Design review of the part built by this model. Coordinates are the model's own, in mm. Coordinates: 2 decimals unless noted, no trailing zeros. Loops run counter-clockwise (first coordinate to the right, second up) from the corner with the lowest first, then second, coordinate; pieces in that order, holes last. Notation, with made-up numbers: (74, -6.75) -> (133, -6.75) arc R23 ccw to (133, 31.25) -> close; hole circle Ø6 at (19, 37.5). An arc over 180 degrees is marked (long way). Answer as a JSON object with one key per item and string values.
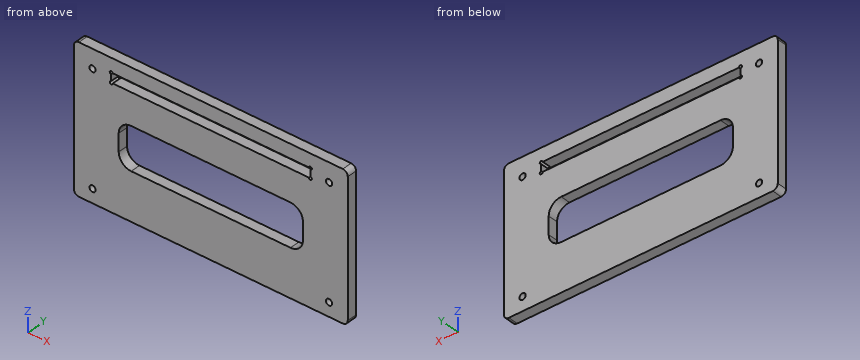
Autodesk Inventor part; units mm, degrees
ref_plane "YZ Plane" through (0, 0, 0) normal (1, 0, 0) x (0, 1, 0)
ref_plane "XZ Plane" through (0, 0, 0) normal (0, 1, 0) x (-1, 0, 0)
ref_plane "XY Plane" through (0, 0, 0) normal (0, 0, 1) x (1, 0, 0)
sketch "Sketch1" plane through (0, 0, 0) normal (0, 1, 0) x (-1, 0, 0)
  line L0 (55, -28) -> (-55, -28)
  line L1 (-55, -28) -> (-55, 28)
  line L2 (-55, 28) -> (55, 28) construction
  line L3 (55, 28) -> (55, -28)
  circle A0 centre (47.5, -22.5) radius 1.25
  circle A1 centre (-47.5, -22.5) radius 1.25
  circle A2 centre (-47.5, 22.5) radius 1.25
  circle A3 centre (47.5, 22.5) radius 1.25
  line L4 (47.5, -22.5) -> (-47.5, -22.5) construction
  line L5 (-47.5, -22.5) -> (-47.5, 22.5) construction
  line L6 (-32, -9) -> (32, -9)
  line L7 (32, 8) -> (-32, 8)
  line L8 (-55, 28) -> (-55, 30)
  line L9 (-55, 30) -> (55, 30)
  line L10 (55, 30) -> (55, 28)
  line L11 (37, 3) -> (37, -4)
  line L12 (-37, 3) -> (-37, -4)
  arc A4 (37, 3) -> (32, 8) centre (32, 3) ccw
  arc A5 (32, -9) -> (37, -4) centre (32, -4) ccw
  arc A6 (-32, 8) -> (-37, 3) centre (-32, 3) ccw
  arc A7 (-37, -4) -> (-32, -9) centre (-32, -4) ccw
  point P0 (0, 0)
  point P1 (-55, 0)
  point P2 (0, 28)
  point P3 (-47.5, 0)
  point P4 (0, -22.5)
  point P5 (-37, -9)
  point P6 (37, -9)
  point P7 (37, 8)
  point P8 (-37, 8)
  point P9 (0, 8)
  dimension "d0" = 110
  dimension "d1" = 56
  dimension "d2" = 2.5
  dimension "d3" = 95
  dimension "d4" = 45
  dimension "d18" = 2
  dimension "d20" = 74
  dimension "d21" = 19
  dimension "d22" = 17
  dimension "d23" = 5
extrude "Extrusion1" add sketch "Sketch1" along normal mid plane 4
fillet "Fillet1" radius 2 4 edges at (55, 0, -28) (-55, 0, -28) (-55, 0, 30) (55, 0, 30)
sketch "Sketch2" plane through (0, 2, 0) normal (0, 1, 0) x (1, 0, 0)
  line L0 (-40, -20.65) -> (-39.4, -20.65) construction
  line L1 (40, -20.65) -> (40, -21.25) construction
  line L2 (40, -24.45) -> (39.4, -24.45) construction
  line L3 (-40, -24.45) -> (-40, -23.85) construction
  arc A0 (-40, -23.85) -> (-39.4, -24.45) centre (-40, -24.45) ccw
  arc A1 (-39.4, -20.65) -> (-40, -21.25) centre (-40, -20.65) ccw
  arc A2 (40, -21.25) -> (39.4, -20.65) centre (40, -20.65) ccw
  arc A3 (39.4, -24.45) -> (40, -23.85) centre (40, -24.45) ccw
  line L4 (-40, -23.85) -> (-40, -21.25)
  line L5 (-39.4, -24.45) -> (-40, -24.45) construction
  arc A4 (-40, -21.25) -> (-39.4, -20.65) centre (-40, -20.65) ccw construction
  line L6 (-40, -21.25) -> (-40, -20.65) construction
  line L7 (-39.4, -20.65) -> (39.4, -20.65)
  line L8 (39.4, -24.45) -> (-39.4, -24.45)
  line L9 (40, -23.85) -> (40, -24.45) construction
  arc A5 (40, -23.85) -> (39.4, -24.45) centre (40, -24.45) ccw construction
  arc A6 (39.4, -20.65) -> (40, -21.25) centre (40, -20.65) ccw construction
  line L10 (40, -21.25) -> (40, -23.85)
  line L11 (39.4, -20.65) -> (40, -20.65) construction
  line L12 (-53, -30) -> (53, -30)
  point P0 (0, 0)
  point P1 (0, -24.45)
  dimension "d9" = 3.8
  dimension "d11" = 80
  dimension "d14" = 1.2
  dimension "d19" = 5.55
extrude "Extrusion2" cut sketch "Sketch2" against normal through all
properties part number "Marco conectores IC DC" material "Polycarbonate, Smoke"
1) Add section C-C, the plane z = 22.5. Give the boundary of the cut face in (x, y), and give its area (3 significant figures).
Completed:
{"outline": "(-55, -2) -> (-48.75, -2) -> (-48.75, 2) -> (-55, 2) -> close; (-46.25, -2) -> (-40, -2) -> (-40, 2) -> (-46.25, 2) -> close; (40, -2) -> (46.25, -2) -> (46.25, 2) -> (40, 2) -> close; (48.75, -2) -> (55, -2) -> (55, 2) -> (48.75, 2) -> close", "area": "100 mm²"}
2) Wall thickness on probe 1 along Z at (x, y) = (-47.5, -0.1); probe 2 along Z at (x, y) = (28.5, 0.95); probe 3 along X at (y, z) = (-1.15, 0.5): over which ranges is each line inside the solid? List them lowest first.
Completed:
{"probe 1": "-28 to -23.75, -21.25 to 21.25, 23.75 to 30", "probe 2": "-28 to -9, 8 to 20.65, 24.45 to 30", "probe 3": "-55 to -37, 37 to 55"}
3) Add section D-D, the plane y = 0.9. Give the boundary of the cut face in (x, z), and give its area (3 significant figures).
Completed:
{"outline": "(-55, -26) arc R2 ccw to (-53, -28) -> (53, -28) arc R2 ccw to (55, -26) -> (55, 28) arc R2 ccw to (53, 30) -> (-53, 30) arc R2 ccw to (-55, 28) -> close; hole circle Ø2.5 at (-47.5, -22.5); hole circle Ø2.5 at (-47.5, 22.5); hole (-40, 21.25) arc R0.6 ccw (long way) to (-39.4, 20.65) -> (39.4, 20.65) arc R0.6 ccw (long way) to (40, 21.25) -> (40, 23.85) arc R0.6 ccw (long way) to (39.4, 24.45) -> (-39.4, 24.45) arc R0.6 ccw (long way) to (-40, 23.85) -> close; hole (-37, -4) arc R5 ccw to (-32, -9) -> (32, -9) arc R5 ccw to (37, -4) -> (37, 3) arc R5 ccw to (32, 8) -> (-32, 8) arc R5 ccw to (-37, 3) -> close; hole circle Ø2.5 at (47.5, -22.5); hole circle Ø2.5 at (47.5, 22.5)", "area": "4,810 mm²"}
4) Add section A-A, the plane z = -1. Give the boundary of the cut face in (x, y).
Completed:
{"outline": "(-55, -2) -> (-37, -2) -> (-37, 2) -> (-55, 2) -> close; (37, -2) -> (55, -2) -> (55, 2) -> (37, 2) -> close"}
5) Add section B-B, the plane x = 16.5. Give the boundary of the cut face in (y, z), and give its area (3 significant figures).
Completed:
{"outline": "(-2, -28) -> (2, -28) -> (2, -9) -> (-2, -9) -> close; (-2, 8) -> (2, 8) -> (2, 20.65) -> (-2, 20.65) -> close; (-2, 24.45) -> (2, 24.45) -> (2, 30) -> (-2, 30) -> close", "area": "149 mm²"}
